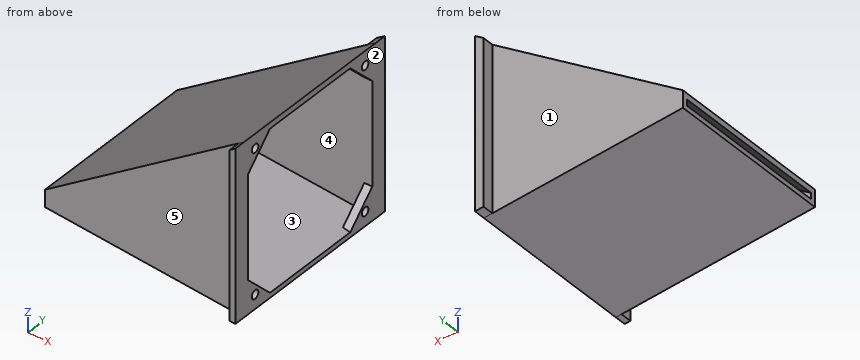
```python
from build123d import *

# Parameters (mm, degrees)
F1_DEPTH  = 60
F2_T      = -1.75
F4_DEPTH  = 2.8
F5_R      = 1.5
F6_DEPTH  = 3
F8_DEPTH  = 4
F10_DEPTH = 4


with BuildPart() as f1:
    # F0 (on Front) → F1 (new body)
    with BuildSketch(Plane.XZ):
        Polygon((0, 50), (-70, 3), (-70, -3), (0, -10), align=None)
    extrude(amount=F1_DEPTH)

    # F2
    f2_openings = [f1.faces().sort_by_distance(p)[0] for p in [
        (0, -30, 20),
        (-70, -30, 0),
    ]]
    offset(amount=F2_T, openings=f2_openings)

    # F3 (on face) → F4 (join)
    with BuildSketch(Plane.YZ):
        Polygon((-58.25, 37.892128), (-48.25, 47.892128), (-58.25, 47.892128), align=None)
        Polygon((-1.75, 47.892128), (-11.75, 47.892128), (-1.75, 37.892128), align=None)
        Polygon((-48.25, -8.241272), (-58.25, 1.758728), (-58.25, -8.241272), align=None)
        Polygon((-1.75, 1.758728), (-11.75, -8.241272), (-1.75, -8.241272), align=None)
    extrude(amount=-F4_DEPTH)

    # F5 (on face) → F6 (cut)
    with BuildSketch(Plane.YZ):
        with Locations((-55, 45)):
            Circle(F5_R)
        with Locations((-5, 45)):
            Circle(F5_R)
        with Locations((-55, -5)):
            Circle(F5_R)
        with Locations((-5, -5)):
            Circle(F5_R)
    extrude(amount=-F6_DEPTH, mode=Mode.SUBTRACT)

    # F7 (on face) → F8 (join)
    with BuildSketch(Plane.XZ.offset(60)):
        Polygon((0, 50), (-1.990074, 48.663807), (-1.990074, -9.800993), (0, -10), align=None)
    extrude(amount=F8_DEPTH)

    # F9 (on face) → F10 (join)
    with BuildSketch(Plane(origin=(0, 0, 0), x_dir=(-1, 0, 0), z_dir=(0, 1, 0))):
        Polygon((2.985112, -9.701489), (2.985112, 47.995711), (0, 50), (0, -10), align=None)
    extrude(amount=F10_DEPTH)


solid = f1.part
```
CAD build for the part. Positions are in the model's coordinates, mm. Face numbers are marked on the shaded views. A direction names the side the tool comes from. Coordinates: 2 decimals unless noted, no trailing zeros. Loops run counter-clockwise (first coordinate to the right, second up) from the corner with the lowest first, then second, coordinate; pieces in that order, holes last. Notation, with made-up numbers: (61, 33.5) - (83, 33.5) arc R6 cw to (83, 40.5) - close; hole circle Ø11 at (19, 13.5). An arc over 180 degrees is marked (long way). Use CSV: the item, a comma, the result in double quotes. Start each with the question number.
Q1. Two-plate mould, pull along Z, no slides. Class the marked faces 3, 4 and 5: +Z half, -Z half, draft (parallel to the pull), parting line (faces both ways), or undercut.
Q2. 3-axis set-ups, long thin cutter, end or side, ignore diameter. For the marked faces 1 and 2: which of +Z, -Z, +X, -X, +Y, -Y reach the whole face in a straight line?
Q3. Probe probe 1 along Y at (x, z) = (-27, 19); probe 2 along Y at (x, z) = (-1.6, 45); probe 3 along Z at (x, y) = (-2.4, -5). List the from-to ranges inside material, lowest first. Write a range as from..to.
Q4. Cut at A-A, the plane y = -37. List the corners of the cut face in (x, z).
Q5. Drop flat-ended pins along their axis: P1, Ø2.5, axis at y = -55, z = 45, coming from the -X side; P2, Ø2.5, axis at y = -5, z = 45, coming from the +X side; P3, Ø6, axis at x = -19, z = 14.5, coming from the -Y side. Give the stop position or say it passes through.
Q6. Cut at B-B, the plane x = -64. List the corners of the cut face in (y, z).
Q7. Cut at C-C, the plane z = -5. List the corners of the cut face in (x, y), then the cut area to 3 significant figures.
Q8. Cut at D-D, the plane y = -5. List the corners of the cut face in (x, z).
Here are the results:
1,face 3,"undercut"
1,face 4,"undercut"
1,face 5,"draft"
2,face 1,"+Z, -Z, -X, +Y"
2,face 2,"+Z, -Z, +X, +Y, -Y"
3,probe 1,"-60..-58.25, -1.75..0"
3,probe 2,"-64..-56.5, -53.5..-51.14, -8.86..-6.5, -3.5..4"
3,probe 3,"-9.76..-6.5, -3.5..-1.49, 41.14..43.5, 46.5..48.39"
4,outline,"(-70, -3) - (0, -10) - (0, -8.24) - (-70, -1.24) - close; (-70, 0.89) - (0, 47.89) - (0, 50) - (-70, 3) - close"
5,P1,"x = -9.31"
5,P2,"x = -3"
5,P3,"y = -60"
6,outline,"(-60, -3.6) - (0, -3.6) - (0, 7.03) - (-60, 7.03) - close; hole (-58.25, -1.84) - (-1.75, -1.84) - (-1.75, 4.92) - (-58.25, 4.92) - close"
7,outline,"(-50, -60) - (-1.99, -60) - (-1.99, -64) - (0, -64) - (0, -56.5) - (-2.8, -56.5) - (-2.8, -58.25) - (-32.41, -58.25) - (-32.41, -1.75) - (-2.8, -1.75) - (-2.8, -3.5) - (0, -3.5) - (0, 4) - (-2.99, 4) - (-2.99, 0) - (-50, 0) - close; (-2.8, -53.5) - (0, -53.5) - (0, -51.49) - (-2.8, -51.49) - close; (-2.8, -8.51) - (0, -8.51) - (0, -6.5) - (-2.8, -6.5) - close"
7,area,"1,210 mm2"
8,outline,"(-70, -3) - (0, -10) - (0, -6.5) - (-2.8, -6.5) - (-2.8, -7.96) - (-70, -1.24) - close; (-70, 0.89) - (-3, 45.88) - (-3, 46.5) - (0, 46.5) - (0, 50) - (-70, 3) - close; (-2.8, -3.5) - (0, -3.5) - (0, -1.49) - (-2.8, -1.49) - close; (-2.8, 41.14) - (0, 41.14) - (0, 43.5) - (-2.8, 43.5) - close"
